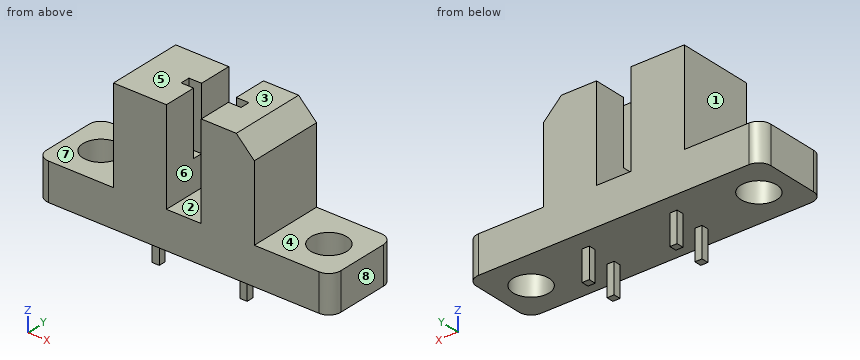
```python
from build123d import *

# Parameters (mm, degrees)
ESBO_O1_W                 = 24.55
ESBO_O1_H                 = 6.35
ESBO_O1_R                 = 1.5
RESSALTO_EXTRUS_O1_DEPTH  = 3.1
ESBO_O2_W                 = 11.75
ESBO_O2_H                 = 6.35
RESSALTO_EXTRUS_O2_DEPTH  = 7.8
ESBO_O5_W                 = 5
ESBO_O5_H                 = 0.8
CORTE_EXTRUS_O2_DEPTH     = 5.25
ESBO_O3_W                 = 2.9
ESBO_O3_H                 = 6.35
CORTE_EXTRUS_O1_DEPTH     = 7.8
CHANFRO3_SIZE             = 1.5
FILETE1_R                 = 1
ESBO_O9_W                 = 0.6
ESBO_O9_H                 = 0.6
RESSALTO_EXTRUS_O3_DEPTH  = 2.5
ESPELHAR2_COPY_1_SKETCH_W = 0.6
ESPELHAR2_COPY_1_SKETCH_H = 0.6
ESPELHAR2_COPY_1_DEPTH    = 2.5


with BuildPart() as part:
    # Esboço1 → Ressalto-extrusão1 (new body)
    with BuildSketch(Plane.XY):
        Rectangle(ESBO_O1_W, ESBO_O1_H)
        with Locations((-9.5, 0)):
            Circle(ESBO_O1_R, mode=Mode.SUBTRACT)
        with Locations((9.5, 0)):
            Circle(ESBO_O1_R, mode=Mode.SUBTRACT)
    extrude(amount=RESSALTO_EXTRUS_O1_DEPTH)

    # Esboço2 → Ressalto-extrusão2 (add)
    with BuildSketch(Plane.XY.offset(3.1)):
        Rectangle(ESBO_O2_W, ESBO_O2_H)
    extrude(amount=RESSALTO_EXTRUS_O2_DEPTH)

    # Esboço5 → Corte-extrusão2 (cut)
    with BuildSketch(Plane.XY.offset(10.9)):
        Rectangle(ESBO_O5_W, ESBO_O5_H)
    extrude(amount=-CORTE_EXTRUS_O2_DEPTH, mode=Mode.SUBTRACT)

    # Esboço3 → Corte-extrusão1 (cut)
    with BuildSketch(Plane.XY.offset(10.9)):
        Rectangle(ESBO_O3_W, ESBO_O3_H)
    extrude(amount=-CORTE_EXTRUS_O1_DEPTH, mode=Mode.SUBTRACT)

    # Chanfro3
    chanfro3_edges = [part.edges().sort_by_distance(p)[0] for p in [
        (5.875, 0, 10.9),
    ]]
    chamfer(chanfro3_edges, length=CHANFRO3_SIZE)

    # Filete1
    filete1_edges = [part.edges().sort_by_distance(p)[0] for p in [
        (12.275, -3.175, 1.55),
        (-12.275, -3.175, 1.55),
        (-12.275, 3.175, 1.55),
        (12.275, 3.175, 1.55),
    ]]
    fillet(filete1_edges, radius=FILETE1_R)

    # Esboço9 → Ressalto-extrusão3 (add)
    with BuildSketch(Plane(origin=(0, 0, 0), x_dir=(-1, 0, 0), z_dir=(0, 0, -1))):
        with Locations((-3.6625, 1.27)):
            Rectangle(ESBO_O9_W, ESBO_O9_H)
    ressalto_extrus_o3 = extrude(amount=RESSALTO_EXTRUS_O3_DEPTH)

    # Espelhar1: Ressalto-extrusão3 across plane
    add(ressalto_extrus_o3.mirror(Plane.ZX))

    # Espelhar2: Ressalto-extrusão3 across plane
    add(ressalto_extrus_o3.mirror(Plane.ZY))

    # Espelhar2 copy 1 sketch → Espelhar2 copy 1 (add)
    with BuildSketch(Plane(origin=(0, 0, 0), x_dir=(1, 0, 0), z_dir=(0, 0, -1))):
        with Locations((-3.6625, 1.27)):
            Rectangle(ESPELHAR2_COPY_1_SKETCH_W, ESPELHAR2_COPY_1_SKETCH_H)
    extrude(amount=ESPELHAR2_COPY_1_DEPTH)


solid = part.part
```
CAD build for the part. Positions are in the model's coordinates, mm. Face numbers are marked on the shaded views. A direction names the side the tool comes from. Give positions to 0.01 mm unless a question says otherwise; leave off trailing zeros. Loops run counter-clockwise (first coordinate to the right, second up) from the corner with the lowest first, then second, coordinate; pieces in that order, holes last. Notation, with made-up numbers: (-30.5, -2) -> (-3.5, -2) arc R18 cw to (-3.5, 13) -> close; hole circle Ø4 at (63.25, 80). An arc over 180 degrees is marked (long way). Use a Markdown table: item, result.
1. Flat gauge pins, fed straight in: pin 1 (2.5 mm diameter, centred on x = 0, y = 1, fed in from +Z); pin 2 (0.7 mm diameter, centred on x = 3.5, z = -1, fed in from +Y); pin 3 (0.7 mm diameter, centred on y = 1, z = -1, fed in from -X); pin 4 (3 mm diameter, centred on x = 4, y = 0.5, fed in from -Z). Where does each tip first touch, or does it go through?
Check result:
| item | result |
|---|---|
| pin 1 | stops at z = 3.1 |
| pin 2 | stops at y = 1.57 |
| pin 3 | stops at x = -3.96 |
| pin 4 | stops at z = -2.5 |
2. Slice it at C-C (y = 0). List the corners of the cut face in (x, z) (3 decimals), plus the area to 3 significant figures.
Check result:
| item | result |
|---|---|
| outline | (-12.275, 0) -> (-11, 0) -> (-11, 3.1) -> (-12.275, 3.1) -> close; (-8, 0) -> (8, 0) -> (8, 3.1) -> (5.875, 3.1) -> (5.875, 9.4) -> (4.375, 10.9) -> (2.5, 10.9) -> (2.5, 5.65) -> (1.45, 5.65) -> (1.45, 3.1) -> (-1.45, 3.1) -> (-1.45, 5.65) -> (-2.5, 5.65) -> (-2.5, 10.9) -> (-5.875, 10.9) -> (-5.875, 3.1) -> (-8, 3.1) -> close; (11, 0) -> (12.275, 0) -> (12.275, 3.1) -> (11, 3.1) -> close |
| area | 114 mm^2 |
3. Slice it at B-B (z = 2.5). List the corners of the cut face in (x, y) (3 decimals).
Check result:
| item | result |
|---|---|
| outline | (-12.275, -2.175) arc R1 ccw to (-11.275, -3.175) -> (11.275, -3.175) arc R1 ccw to (12.275, -2.175) -> (12.275, 2.175) arc R1 ccw to (11.275, 3.175) -> (-11.275, 3.175) arc R1 ccw to (-12.275, 2.175) -> close; hole circle Ø3 at (-9.5, 0); hole circle Ø3 at (9.5, 0) |
4. Which spindle directions (+Z, -Z, +X, -X, +Y, -Y) get a long thin tool onto all of the face, cutting with end or side? Do the marked faces 4, 5, 6, 7 and 8. Say none if no direction does.
Check result:
| item | result |
|---|---|
| face 4 | +Z, +X, +Y, -Y |
| face 5 | +Z, +X, -X, +Y, -Y |
| face 6 | +Z, +Y, -Y |
| face 7 | +Z, -X, +Y, -Y |
| face 8 | +Z, -Z, +X, +Y, -Y |
5. Slice it at A-A (x = -9.5). List the corners of the cut face in (y, z) (3 decimals), plus the area to 3 significant figures.
Check result:
| item | result |
|---|---|
| outline | (-3.175, 0) -> (-1.5, 0) -> (-1.5, 3.1) -> (-3.175, 3.1) -> close; (1.5, 0) -> (3.175, 0) -> (3.175, 3.1) -> (1.5, 3.1) -> close |
| area | 10.4 mm^2 |
6. Slice it at D-D (z = 4.25). List the corners of the cut face in (x, y) (3 decimals).
Check result:
| item | result |
|---|---|
| outline | (-5.875, -3.175) -> (-1.45, -3.175) -> (-1.45, 3.175) -> (-5.875, 3.175) -> close; (1.45, -3.175) -> (5.875, -3.175) -> (5.875, 3.175) -> (1.45, 3.175) -> close |
7. Wall check: L1, parallel to X at y = -2, z = 8.5 (3 decimals); L2, parallel to Y at x = -9.5, z = 0.75 (3 decimals); L3, parallel to X at y = 1.5, z = -1. Give the ranges that are in metal, low to high. Write a range as [from, to].
Check result:
| item | result |
|---|---|
| L1 | x = [-5.875, -1.45], [1.45, 5.875] |
| L2 | y = [-3.175, -1.5], [1.5, 3.175] |
| L3 | x = [-3.96, -3.36], [3.36, 3.96] |
8. Mould opens along X. For the marked faces 1, 2 and 3 say: pulls with the +X half, pulls with the -X half, needs draft (parallel to the pull), parting line crosses it, or undercut.
Check result:
| item | result |
|---|---|
| face 1 | pulls with the -X half |
| face 2 | undercut |
| face 3 | needs draft |
